Can you work these out from the model? Positions are in its coordinate system, mm. A direction names the side the tool comes from. Round coordinates to 2 decimals unless told otherwise and drop trailing zeros. Order: outer loops, then holes, each group sorted by start corner. A loop starts at its lowest first (then second) coordinate and runs counter-clockwise, first axis right, second up. Notation, with made-up numbers: (-25.5, -36) -> (-1.5, -36) arc R16 ccw to (-1.5, -31) -> close; hole circle Ø10 at (-21.5, 89.25). An arc over 180 degrees is marked (long way). Use a Markdown table: item, result. Add a question column.
Q1. I'm going to push flat-ended pins straight in: pin 1 Ø1.5 at (y, z) = (2, 21) entering from -X; pin 2 Ø4 at (x, z) = (40.33, 0) entering from +Y; pin 3 Ø2 at (x, y) = (-7, 4.5) entering from -Z. Where does each tip first touch, or does it pass through?
Q2. If we section it at A-A on x = 0: List the corners of the cut face in (y, z) for me, plus the area to 3 significant figures.
Q3. We'd pull the mould along X, two halves only. Please class faces 1 (the face through (12.864, 6.084, -6.691)), 2 (the face through (-39.953, 14.535, -6.328)), 3 (the face through (-41, 17, -2)): +X half, -X half, draft (parallel to the pull), parting line (faces both ways), or undercut.
Q4. If we section it at C-C on y = 2: List the corners of the cut face in (x, z) for me.
Q5. I need wall thicknesses on line 1 along X through (y, z) = (9.25, 0); line 2 along Y through (x, z) = (-18, 19.5); line 3 along Z through (x, y) = (19, 10). Which ranges of each line are inside material? Lowest first, please. Write a range as [from, to].
Q6. If we section it at B-B on z = -3: List the corners of the cut face in (x, y) for me, plus the area to 3 significant figures.
Q7. If we section it at D-D on x = -9: List the corners of the cut face in (y, z) for me.
Q8. For faces 4 (the face through (-21.64, 6.08, -35.87)), 5 (the face through (-40.05, 14.535, 6.343)), which set-ups out of +Z, -Z, +X, -X, +Y, -Y let a thin tool reach every point of the face, with its end or its side?
```python
from build123d import *

# Parameters (mm, degrees)
SKETCH1_W           = 29.5
SKETCH1_H           = 12
BOSS_EXTRUDE1_START = 5
BOSS_EXTRUDE1_DEPTH = 5
SKETCH3_R           = 1.75
CUT_EXTRUDE1_DEPTH  = 65.505813691
CIRPATTERN1_COUNT   = 6


with BuildPart() as part:
    # Sketch1 → Revolve1 (revolve)
    with BuildSketch(Plane.XY, mode=Mode.PRIVATE) as revolve1_sk:
        with Locations((29.25, 6)):
            Rectangle(SKETCH1_W, SKETCH1_H)
    revolve(revolve1_sk.sketch.rotate(Axis((0, 0, 0), (0, 1, 0)), 90), axis=Axis((0, 0, 0), (0, 1, 0)))

    # Sketch2 → Boss-Extrude1 (add)
    with BuildSketch(Plane(origin=(0, 12, 0), x_dir=(1, 0, 0), z_dir=(0, 1, 0)).offset(BOSS_EXTRUDE1_START)):
        with BuildLine():
            Line((-44, 0), (-37, 0))
            ThreePointArc((-37, 0), (-36.885941348, 2.902986542), (-36.544468602, 5.788075206))
            Line((-36.544468602, 5.788075206), (-43.458286986, 6.883116462))
            ThreePointArc((-43.458286986, 6.883116462), (-43.864362684, 3.452200212), (-44, 0))
        make_face()
        with BuildLine():
            ThreePointArc((-36.544468602, -5.788075206), (-36.885941348, -2.902986542), (-37, 0))
            Line((-37, 0), (-44, 0))
            ThreePointArc((-44, 0), (-43.864362684, -3.452200212), (-43.458286986, -6.883116462))
            Line((-43.458286986, -6.883116462), (-36.544468602, -5.788075206))
        make_face()
    extrude(amount=-BOSS_EXTRUDE1_DEPTH)

    # Sketch3 → Cut-Extrude1 (cut, through all)
    with BuildSketch(Plane(origin=(0, 17, 0), x_dir=(1, 0, 0), z_dir=(0, 1, 0))):
        with Locations(Location((-40.332863527, 0, 0), (0, 0, 270))):
            Circle(SKETCH3_R)
    cut_extrude1 = extrude(amount=-CUT_EXTRUDE1_DEPTH, mode=Mode.SUBTRACT)

    # CirPattern1: Cut-Extrude1 ×6 about axis
    cirpattern1_axis = Axis((0, 0, 0), (0, 1, 0))
    for i in range(1, CIRPATTERN1_COUNT):
        add(cut_extrude1.rotate(cirpattern1_axis, i * 360 / CIRPATTERN1_COUNT), mode=Mode.SUBTRACT)


solid = part.part
```
Answer below:
| question | item | result |
|---|---|---|
| 1 | pin 1 | x = -39.06 |
| 1 | pin 2 | y = 12 |
| 1 | pin 3 | z = -43.59 |
| 2 | outline | (0, -44) -> (12, -44) -> (12, -14.5) -> (0, -14.5) -> close; (0, 14.5) -> (12, 14.5) -> (12, 44) -> (0, 44) -> close |
| 2 | area | 708 mm² |
| 3 | face 1 | undercut |
| 3 | face 2 | +X half |
| 3 | face 3 | draft |
| 4 | outline | circle Ø88 at (0, 0); hole circle Ø3.5 at (-40.33, 0); hole circle Ø3.5 at (-20.17, -34.93); hole circle Ø3.5 at (-20.17, 34.93); hole circle Ø29 at (0, 0); hole circle Ø3.5 at (20.17, -34.93); hole circle Ø3.5 at (20.17, 34.93); hole circle Ø3.5 at (40.33, 0) |
| 5 | line 1 | [-44, -42.08], [-38.58, -14.5], [14.5, 38.58], [42.08, 44] |
| 5 | line 2 | [0, 12] |
| 5 | line 3 | [-39.69, -36.23], [-33.62, 33.62], [36.23, 39.69] |
| 6 | outline | (-43.9, 0) -> (-14.19, 0) -> (-14.19, 12) -> (-36.88, 12) -> (-36.88, 17) -> (-43.9, 17) -> close; (14.19, 0) -> (43.9, 0) -> (43.9, 12) -> (14.19, 12) -> close |
| 6 | area | 748 mm² |
| 7 | outline | (0, -43.07) -> (12, -43.07) -> (12, -11.37) -> (0, -11.37) -> close; (0, 11.37) -> (12, 11.37) -> (12, 43.07) -> (0, 43.07) -> close |
| 8 | face 4 | +Y, -Y |
| 8 | face 5 | +Z, +X, +Y |
